from build123d import *

# Parameters (mm, degrees)
CROQUIS1_W              = 110
CROQUIS1_H              = 15
SALIENTE_EXTRUIR1_DEPTH = 5
REDONDEO1_R             = 3
CROQUIS2_R              = 4
CORTAR_EXTRUIR1_DEPTH   = 56.733742024


with BuildPart() as part:
    # Croquis1 → Saliente-Extruir1 (new body)
    with BuildSketch(Plane(origin=(0, 0, 0), x_dir=(1, 0, 0), z_dir=(0, 1, 0))):
        Rectangle(CROQUIS1_W, CROQUIS1_H)
    extrude(amount=SALIENTE_EXTRUIR1_DEPTH)

    # Redondeo1
    redondeo1_edges = [part.edges().sort_by_distance(p)[0] for p in [
        (55, 2.5, 7.5),
        (-55, 2.5, 7.5),
        (-55, 2.5, -7.5),
        (55, 2.5, -7.5),
    ]]
    fillet(redondeo1_edges, radius=REDONDEO1_R)

    # Croquis2 → Cortar-Extruir1 (cut, through all)
    with BuildSketch(Plane(origin=(0, 5, 0), x_dir=(1, 0, 0), z_dir=(0, 1, 0))):
        with Locations(Location((-47.5, 0, 0), (0, 0, 270))):
            Circle(CROQUIS2_R)
        with Locations(Location((47.5, 0, 0), (0, 0, 270))):
            Circle(CROQUIS2_R)
    extrude(amount=-CORTAR_EXTRUIR1_DEPTH, mode=Mode.SUBTRACT)


solid = part.part
For this review, take the finished solid that the model builds, in its own axes (mm). Round coordinates to 2 decimals unless told otherwise and drop trailing zeros. Loops run counter-clockwise (first coordinate to the right, second up) from the corner with the lowest first, then second, coordinate; pieces in that order, holes last. Notation, with made-up numbers: (88, -11) - (106, -11) arc R19 ccw to (106, 24) - close; hole circle Ø3 at (-13.75, 77). An arc over 180 degrees is marked (long way). Use one line per item in the form item = value.
1) We need section C-C on y = 3.6. Write out the cut boundary in (x, z).
Solutions:
outline = (-55, -4.5) arc R3 ccw to (-52, -7.5) - (52, -7.5) arc R3 ccw to (55, -4.5) - (55, 4.5) arc R3 ccw to (52, 7.5) - (-52, 7.5) arc R3 ccw to (-55, 4.5) - close; hole circle Ø8 at (-47.5, 0); hole circle Ø8 at (47.5, 0)
2) We need section A-A on z = 0. Write out the cut boundary in (x, y), then the cut area to 3 significant figures.
Solutions:
outline = (-55, 0) - (-51.5, 0) - (-51.5, 5) - (-55, 5) - close; (-43.5, 0) - (43.5, 0) - (43.5, 5) - (-43.5, 5) - close; (51.5, 0) - (55, 0) - (55, 5) - (51.5, 5) - close
area = 470 mm2
3) We need section B-B on x = -47.5. Write out the cut boundary in (y, z), then the cut area to 3 significant figures.
Solutions:
outline = (0, -7.5) - (5, -7.5) - (5, -4) - (0, -4) - close; (0, 4) - (5, 4) - (5, 7.5) - (0, 7.5) - close
area = 35.0 mm2
4) Mouldability with a two-part tool opening along X and no side actions: class faces 1 (the face through (-1, 2, 7.5)), 2 (the face through (-54.14, 2.54, 6.6)), 3 (the face through (-43.534, 2.535, -0.521)) as pulls with the +X half, pulls with the -X half, needs draft (parallel to the pull), parting line crosses it, or undercut.
Solutions:
face_1 = needs draft
face_2 = pulls with the -X half
face_3 = undercut
5) Wall thickness on probe 1 along X at (y, z) = (3.4, 0); probe 2 along X at (y, z) = (1, -3); probe 3 along Z at (x, y) = (-44.5, 1.25): over which ranges is each line inside the solid? List them lowest first.
Solutions:
probe_1 = -55 to -51.5, -43.5 to 43.5, 51.5 to 55
probe_2 = -55 to -50.15, -44.85 to 44.85, 50.15 to 55
probe_3 = -7.5 to -2.65, 2.65 to 7.5
